from build123d import *

# Parameters (mm, degrees)
F1_DEPTH = 7.5


with BuildPart() as f1:
    # F0 (on Top) → F1 (new body)
    with BuildSketch(Plane.XY):
        with BuildLine():
            Line((-3.341401, 25.115587), (-12.866401, 25.115587))
            Line((-12.866401, 25.115587), (-12.866401, -44.884413))
            Line((-12.866401, -44.884413), (-3.341401, -44.884413))
            Line((-3.341401, -44.884413), (-3.341401, -41.836413))
            ThreePointArc((-3.341401, -41.836413), (-6.643401, -38.534413), (-3.341401, -35.232413))
            Line((-3.341401, -35.232413), (-3.341401, 25.115587))
        make_face()
        with BuildLine():
            Line((6.183599, 25.115587), (-3.341401, 25.115587))
            Line((-3.341401, 25.115587), (-3.341401, -35.232413))
            ThreePointArc((-3.341401, -35.232413), (-1.006534, -36.199547), (-0.039401, -38.534413))
            ThreePointArc((-0.039401, -38.534413), (-1.006534, -40.86928), (-3.341401, -41.836413))
            Line((-3.341401, -41.836413), (-3.341401, -44.884413))
            Line((-3.341401, -44.884413), (6.183599, -44.884413))
            Line((6.183599, -44.884413), (6.183599, 25.115587))
        make_face()
    extrude(amount=F1_DEPTH)


solid = f1.part
Can you work these out from the model? Positions are in its coordinate system, mm. Round coordinates to 2 decimals unless told otherwise and drop trailing zeros. Write each loop counter-clockwise with the first axis right and the second up, starting at its lowest first coordinate (ties: lowest second). Pieces come first, ordered by that corner, then holes. Notation, with made-up numbers: (-38, 42) -> (-25, 42) arc R18 cw to (-25, 75) -> close; hole circle Ø3 at (-27, -22). An arc over 180 degrees is marked (long way). One line per question, with ' | ' between items. Start each with the question number.
1) I need wall thicknesses on line 1 (Y direction, x = -2, z = 6.5); line 2 (X direction, y = -40.5, z = 3.5); line 3 (Y direction, x = -2.25, z = 5.25). Which ranges of each line are inside material? Lowest first, please. Write a range as [from, to].
2) Suppose I cut it at C-C on x = -0.75. Write out the boundary of the cut face in (y, z), then the cut area to 3 significant figures.
3) Suppose I cut it at A-A on x = -5.75. Write out the boundary of the cut face in (y, z).
4) Suppose I cut it at B-B on z = 2.5. Write out the boundary of the cut face in (x, y), then the cut area to 3 significant figures.
Return value:
1) line 1: y = [-44.88, -41.55], [-35.52, 25.12] | line 2: x = [-12.87, -5.99], [-0.69, 6.18] | line 3: y = [-44.88, -41.65], [-35.42, 25.12]
2) outline: (-44.88, 0) -> (-40.58, 0) -> (-40.58, 7.5) -> (-44.88, 7.5) -> close; (-36.49, 0) -> (25.12, 0) -> (25.12, 7.5) -> (-36.49, 7.5) -> close | area: 494 mm2
3) outline: (-44.88, 0) -> (-40.79, 0) -> (-40.79, 7.5) -> (-44.88, 7.5) -> close; (-36.28, 0) -> (25.12, 0) -> (25.12, 7.5) -> (-36.28, 7.5) -> close
4) outline: (-12.87, -44.88) -> (6.18, -44.88) -> (6.18, 25.12) -> (-12.87, 25.12) -> close; hole (-3.34, -41.84) arc R3.3 ccw to (-0.04, -38.53) arc R3.3 ccw (long way) to start | area: 1,300 mm2
